from build123d import *

# Parameters (mm, degrees)
SKETCH1_R           = 35
BOSS_EXTRUDE1_DEPTH = 5
SKETCH3_R           = 37.5
BOSS_EXTRUDE2_DEPTH = 5
SKETCH4_R           = 27.5
BOSS_EXTRUDE5_DEPTH = 104.5
SKETCH5_R           = 32.5
BOSS_EXTRUDE6_DEPTH = 5
SKETCH6_R           = 30
BOSS_EXTRUDE7_DEPTH = 3
FILLET1_R           = 10
FILLET2_R           = 10


# Read off the part's stored shape, not the designer's step: Shell1
with BuildPart() as part:
    # Sketch1 → Boss-Extrude1 (new body)
    with BuildSketch(Plane(origin=(0, 0, 0), x_dir=(1, 0, 0), z_dir=(0, 1, 0))):
        with Locations(Location((0, 0, 0), (0, 0, 270))):
            Circle(SKETCH1_R)
    extrude(amount=BOSS_EXTRUDE1_DEPTH)

    # Sketch3 → Boss-Extrude2 (add)
    with BuildSketch(Plane(origin=(0, 5, 0), x_dir=(1, 0, 0), z_dir=(0, 1, 0))):
        with Locations(Location((0, 0, 0), (0, 0, 270))):
            Circle(SKETCH3_R)
    extrude(amount=BOSS_EXTRUDE2_DEPTH)

    # Sketch4 → Boss-Extrude5 (add)
    with BuildSketch(Plane(origin=(0, 10, 0), x_dir=(1, 0, 0), z_dir=(0, 1, 0))):
        with Locations(Location((0, 0, 0), (0, 0, 270))):
            Circle(SKETCH4_R)
    extrude(amount=BOSS_EXTRUDE5_DEPTH)

    # Sketch5 → Boss-Extrude6 (add)
    with BuildSketch(Plane(origin=(0, 114.5, 0), x_dir=(1, 0, 0), z_dir=(0, 1, 0))):
        with Locations(Location((0, 0, 0), (0, 0, 270))):
            Circle(SKETCH5_R)
    extrude(amount=BOSS_EXTRUDE6_DEPTH)

    # Sketch6 → Boss-Extrude7 (add)
    with BuildSketch(Plane(origin=(0, 119.5, 0), x_dir=(1, 0, 0), z_dir=(0, 1, 0))):
        with Locations(Location((0, 0, 0), (0, 0, 270))):
            Circle(SKETCH6_R)
    extrude(amount=BOSS_EXTRUDE7_DEPTH)

    # Fillet1
    # the kernel refuses this fillet: 10 mm, written as the material it adds along each edge
    with BuildSketch(Plane(origin=(0, 10, 0), x_dir=(0, 0, 1), z_dir=(-1, 0, 0))) as fillet1_piece_1:
        with BuildLine():
            CenterArc((27.5 + FILLET1_R, FILLET1_R), FILLET1_R, 180, 90)
            Line((27.5 + FILLET1_R, 0), (27.5 + FILLET1_R, -FILLET1_R * 0.02))
            Line((27.5 + FILLET1_R, -FILLET1_R * 0.02), (27.5 - FILLET1_R * 0.02, -FILLET1_R * 0.02))
            Line((27.5 - FILLET1_R * 0.02, -FILLET1_R * 0.02), (27.5 - FILLET1_R * 0.02, FILLET1_R))
            Line((27.5 - FILLET1_R * 0.02, FILLET1_R), (27.5, FILLET1_R))
        make_face()
    revolve(axis=Axis((0, 10, 0), (0, 1, 0)))
    with BuildSketch(Plane(origin=(0, 114.5, 0), x_dir=(0, 0, 1), z_dir=(-1, 0, 0))) as fillet1_piece_2:
        with BuildLine():
            CenterArc((37.5, -8.660254038), FILLET1_R, 120, 60)
            Line((27.5, -8.660254038), (27.3, -8.660254038))
            Line((27.3, -8.660254038), (27.3, 0))
            Line((27.3, 0), (27.5, 0.2))
            ThreePointArc((27.5, 0.2), (30, 0.2), (32.4, 0.173205081))
            Line((32.4, 0.173205081), (32.5, 0))
        make_face()
    revolve(axis=Axis((0, 114.5, 0), (0, 1, 0)))

    # Fillet2
    # the kernel refuses this fillet: 10 mm, written as the material it takes off along each edge
    with BuildSketch(Plane(origin=(0, 114.5, 0), x_dir=(0, 0, 1), z_dir=(-1, 0, 0))) as fillet2_piece_1:
        with BuildLine():
            CenterArc((22.5, 4.568502517), FILLET2_R, 318.590377891, 41.409622109)
            Line((32.5, 4.568502517), (32.7, 4.568502517))
            Line((32.7, 4.568502517), (32.7, 0))
            Line((32.7, 0), (32.6, -0.173205081))
            ThreePointArc((32.6, -0.173205081), (31.293504258, -1.076098804), (30.15, -2.178163326))
            Line((30.15, -2.178163326), (30, -2.04587576))
        make_face()
    revolve(axis=Axis((0, 114.5, 0), (0, 1, 0)), mode=Mode.SUBTRACT)
    with BuildSketch(Plane(origin=(0, 10, 0), x_dir=(0, 0, 1), z_dir=(-1, 0, 0))) as fillet2_piece_2:
        with BuildLine():
            CenterArc((27.817541634, -7.5), FILLET2_R, 14.477512186, 46.567463442)
            Line((37.5, -5), (37.693649167, -4.95))
            ThreePointArc((37.693649167, -4.95), (37.7, -2.5), (37.7, 0))
            Line((37.7, 0), (37.5, 0.2))
            ThreePointArc((37.5, 0.2), (35.05, 0.511190802), (32.755595401, 1.425))
            Line((32.755595401, 1.425), (32.658770817, 1.25))
        make_face()
    revolve(axis=Axis((0, 10, 0), (0, 1, 0)), mode=Mode.SUBTRACT)

    # Shell1 outline → Shell1 (revolve, cut)
    with BuildSketch(Plane.XY):
        with BuildLine():
            ThreePointArc((28.125, 114.107718809), (29.07798837, 115.465716235), (29.709112104, 117))
            Line((29.709112104, 117), (27.5, 117))
            Line((27.5, 117), (27.5, 122.5))
            Line((27.5, 122.5), (0, 122.5))
            Line((0, 122.5), (0, 0))
            Line((0, 0), (32.5, 0))
            Line((32.5, 0), (32.5, 7.5))
            Line((32.5, 7.5), (33.407711578, 7.5))
            ThreePointArc((33.407711578, 7.5), (32.493809933, 8.363660529), (31.448463522, 9.0625))
            ThreePointArc((31.448463522, 9.0625), (26.732126348, 13.65154373), (25, 20))
            Line((25, 20), (25, 105.839745962))
            ThreePointArc((25, 105.839745962), (25.807320666, 110.259163345), (28.125, 114.107718809))
        make_face()
    revolve(axis=Axis((0, 0, 0), (0, 1, 0)), mode=Mode.SUBTRACT)


solid = part.part
Input: part model. Units: mm. Frame: model coordinates. A direction names the side the tool comes from. Coordinates: 2 decimals unless noted, no trailing zeros. Loops run counter-clockwise (first coordinate to the right, second up) from the corner with the lowest first, then second, coordinate; pieces in that order, holes last.
Q1. Cut plane A-A (y = 88). Output: boundary loops of the cut face in (x, z), then the cut area to 3 significant figures.
Q2. Draft query along Z for faces 1 (the face through (-7, 7.5, 32)), 2 (the face through (-23.2, 0, 23.2)), 3 (the face through (1.32, 120.98, -29.97)). Return one class per face: +Z half, -Z half, draft (parallel to the pull), parting line (faces both ways), or undercut.
Q3. Material intervals for line 1 (X direction, y = 119.35, z = 0); line 2 (X direction, y = 120.05, z = 0); line 3 (Z direction, x = -5, y = 113), sorted ascending.
Q4. Set-up query: faces 4 (the face through (-21, 2, -28)), 5 (the face through (-29, 119.5, 9)), 6 (the face through (-24.397, 62.319, 12.69)). Return all of +Z, -Z, +X, -X, +Y, -Y with unobstructed straight access to the full face (end or side cutting, diameter ignored); none if empty.
Q5. Contact query for flat-ended pins moving along their axis: pin 1 (2 mm diameter, centred on y = 34.5, z = -8.5, fed in from +X); pin 2 (10 mm diameter, centred on x = -24.5, z = 4, fed in from -Y); pin 3 (2 mm diameter, centred on x = 13.5, y = 109, fed in from -Z). Output: stop coordinate, or through.
Working result:
1. outline: circle Ø55 at (0, 0); hole circle Ø50 at (0, 0)
1. area: 412 mm2
2. face 1: undercut
2. face 2: draft
2. face 3: parting line
3. line 1: x = -32.5 to -27.5, 27.5 to 32.5
3. line 2: x = -30 to -27.5, 27.5 to 30
3. line 3: z = -30.03 to -26.79, 26.79 to 30.03
4. face 4: -Y
4. face 5: +Y
4. face 6: none
5. pin 1: stops at x = 26.46
5. pin 2: stops at y = 10.13
5. pin 3: stops at z = -25.22
